```python
from build123d import *

# Parameters (mm, degrees)
SKETCH1_W            = 24.13
SKETCH1_H            = 10.16
BOSS_EXTRUDE1_DEPTH  = 5.334
SKETCH6_W            = 5.334
SKETCH6_H            = 10.16
BOSS_EXTRUDE5_DEPTH  = 5.334
SKETCH11_W           = 5.334
SKETCH11_H           = 10.206206115
BOSS_EXTRUDE6_DEPTH  = 5.334
SKETCH12_W           = 34.798
SKETCH12_H           = 5.334
BOSS_EXTRUDE7_DEPTH  = 5.334
SKETCH13_W           = 5.334
SKETCH13_H           = 0.046206115
CUT_EXTRUDE1_DEPTH   = 32.634561721
SKETCH17_W           = 11.599333333
SKETCH17_H           = 5.334
CUT_EXTRUDE5_DEPTH   = 5.334
SKETCH18_W           = 5.334
SKETCH18_H           = 5.08
SKETCH18_W_2         = 11.684
CUT_EXTRUDE6_DEPTH   = 5.334
SKETCH19_W           = 5.334
SKETCH19_H           = 5.08
BOSS_EXTRUDE8_DEPTH  = 5.334
SKETCH20_W           = 5.334
SKETCH20_H           = 5.08
BOSS_EXTRUDE10_DEPTH = 1.016
SKETCH21_W           = 11.599333334
SKETCH21_H           = 5.334
BOSS_EXTRUDE11_DEPTH = 10.668
SKETCH22_W           = 5.503333334
SKETCH22_H           = 5.334
CUT_EXTRUDE7_DEPTH   = 34.950594339
SKETCH23_W           = 5.334
SKETCH23_H           = 5.08
BOSS_EXTRUDE12_DEPTH = 5.334
SKETCH24_W           = 5.334
SKETCH24_H           = 5.08
CUT_EXTRUDE8_DEPTH   = 5.334
SKETCH25_W           = 5.334
SKETCH25_H           = 5.08
BOSS_EXTRUDE13_DEPTH = 5.334
SKETCH26_W           = 5.334
SKETCH26_H           = 5.08
CUT_EXTRUDE9_DEPTH   = 5.334


with BuildPart() as part:
    # Sketch1 → Boss-Extrude1 (new body)
    with BuildSketch(Plane.XY):
        with Locations((12.065, 5.08)):
            Rectangle(SKETCH1_W, SKETCH1_H)
    extrude(amount=BOSS_EXTRUDE1_DEPTH)

    # Sketch6 → Boss-Extrude5 (add)
    with BuildSketch(Plane(origin=(24.13, 0, 0), x_dir=(0, 0, -1), z_dir=(1, 0, 0))):
        with Locations((-2.667, 5.08)):
            Rectangle(SKETCH6_W, SKETCH6_H)
    extrude(amount=BOSS_EXTRUDE5_DEPTH)

    # Sketch11 → Boss-Extrude6 (add)
    with BuildSketch(Plane.ZY):
        with Locations((2.667, 5.103103058)):
            Rectangle(SKETCH11_W, SKETCH11_H)
    extrude(amount=BOSS_EXTRUDE6_DEPTH)

    # Sketch12 → Boss-Extrude7 (add)
    with BuildSketch(Plane(origin=(0, 0, 0), x_dir=(-1, 0, 0), z_dir=(0, -1, 0))):
        with Locations((-12.065, -2.667)):
            Rectangle(SKETCH12_W, SKETCH12_H)
    extrude(amount=BOSS_EXTRUDE7_DEPTH)

    # Sketch13 → Cut-Extrude1 (cut, through all)
    with BuildSketch(Plane(origin=(0, 0, 0), x_dir=(-1, 0, 0), z_dir=(0, 0, -1))):
        with Locations((2.667, 10.183103058)):
            Rectangle(SKETCH13_W, SKETCH13_H)
    extrude(amount=-CUT_EXTRUDE1_DEPTH, mode=Mode.SUBTRACT)

    # Sketch17 → Cut-Extrude5 (cut)
    with BuildSketch(Plane(origin=(0, -5.334, 0), x_dir=(-1, 0, 0), z_dir=(0, -1, 0))):
        with Locations((-0.465666666, -2.667)):
            Rectangle(SKETCH17_W, SKETCH17_H)
        with Locations((-23.664333334, -2.667)):
            Rectangle(SKETCH17_W, SKETCH17_H)
    extrude(amount=-CUT_EXTRUDE5_DEPTH, mode=Mode.SUBTRACT)

    # Sketch18 → Cut-Extrude6 (cut)
    with BuildSketch(Plane.XY.offset(5.334)):
        with Locations((-2.667, 7.62)):
            Rectangle(SKETCH18_W, SKETCH18_H)
        with Locations((23.622, 7.62)):
            Rectangle(SKETCH18_W_2, SKETCH18_H)
    extrude(amount=-CUT_EXTRUDE6_DEPTH, mode=Mode.SUBTRACT)

    # Sketch19 → Boss-Extrude8 (add)
    with BuildSketch(Plane(origin=(17.78, 0, 0), x_dir=(0, 0, -1), z_dir=(1, 0, 0))):
        with Locations((-2.667, 7.62)):
            Rectangle(SKETCH19_W, SKETCH19_H)
    extrude(amount=BOSS_EXTRUDE8_DEPTH)

    # Sketch20 → Boss-Extrude10 (add)
    with BuildSketch(Plane(origin=(23.114, 0, 0), x_dir=(0, 0, -1), z_dir=(1, 0, 0))):
        with Locations((-2.667, 7.62)):
            Rectangle(SKETCH20_W, SKETCH20_H)
    extrude(amount=BOSS_EXTRUDE10_DEPTH)

    # Sketch21 → Boss-Extrude11 (add)
    with BuildSketch(Plane.XZ.offset(5.334)):
        with Locations((12.065, 2.667)):
            Rectangle(SKETCH21_W, SKETCH21_H)
    extrude(amount=BOSS_EXTRUDE11_DEPTH)

    # Sketch22 → Cut-Extrude7 (cut, through all)
    with BuildSketch(Plane.XY.offset(5.334)):
        with Locations((12.065, -8.001)):
            Rectangle(SKETCH22_W, SKETCH22_H)
    extrude(amount=-CUT_EXTRUDE7_DEPTH, mode=Mode.SUBTRACT)

    # Sketch23 → Boss-Extrude12 (add)
    with BuildSketch(Plane.ZY):
        with Locations((2.667, 7.62)):
            Rectangle(SKETCH23_W, SKETCH23_H)
    extrude(amount=BOSS_EXTRUDE12_DEPTH)

    # Sketch24 → Cut-Extrude8 (cut)
    with BuildSketch(Plane.ZY.offset(5.334)):
        with Locations((2.667, 2.54)):
            Rectangle(SKETCH24_W, SKETCH24_H)
    extrude(amount=-CUT_EXTRUDE8_DEPTH, mode=Mode.SUBTRACT)

    # Sketch25 → Boss-Extrude13 (add)
    with BuildSketch(Plane(origin=(24.13, 0, 0), x_dir=(0, 0, -1), z_dir=(1, 0, 0))):
        with Locations((-2.667, 7.62)):
            Rectangle(SKETCH25_W, SKETCH25_H)
    extrude(amount=BOSS_EXTRUDE13_DEPTH)

    # Sketch26 → Cut-Extrude9 (cut)
    with BuildSketch(Plane(origin=(29.464, 0, 0), x_dir=(0, 0, -1), z_dir=(1, 0, 0))):
        with Locations((-2.667, 2.54)):
            Rectangle(SKETCH26_W, SKETCH26_H)
    extrude(amount=-CUT_EXTRUDE9_DEPTH, mode=Mode.SUBTRACT)


solid = part.part
```
Part model, mm, in its own coordinate system. A direction names the side the tool comes from. Give positions to 0.01 mm unless a question says otherwise; leave off trailing zeros. Loops run counter-clockwise (first coordinate to the right, second up) from the corner with the lowest first, then second, coordinate; pieces in that order, holes last. Notation, with made-up numbers: M 2,32 L 55,32 A21 cw 55,36 Z; hole C -20.5,22 d9. An arc over 180 degrees is marked long. Return JSON: item names as keys, results as strings.
1) 3-axis set-ups, long thin cutter, end or side, ignore diameter. For faces 1 (the face through (9.313, -8, 3)), 2 (the face through (17.865, -8, 3)), 3 (the face through (6.265, -8, 3)): which of +Z, -Z, +X, -X, +Y, -Y reach the whole face in a straight line?
Calculated:
{"face 1": "+Z, -Z", "face 2": "+Z, -Z, +X, -Y", "face 3": "+Z, -Z, -X, -Y"}
2) Drill centre lines: line 1 (X direction, y = -7.5, z = 3); line 2 (Y direction, x = 4.5, z = 1.55); line 3 (X direction, y = -0.75, z = 4.6). Where is each one in solid material? Low to high.
Calculated:
{"line 1": "x = 6.27 to 9.31, 14.82 to 17.86", "line 2": "y = 0 to 10.16", "line 3": "x = 6.27 to 17.86"}
3) Saw through at B-B, the plane y = -8.75. List the corners of the cut face in (x, z), then the cut area to 3 significant figures.
Calculated:
{"outline": "M 6.27,0 L 9.31,0 L 9.31,5.33 L 6.27,5.33 Z; M 14.82,0 L 17.86,0 L 17.86,5.33 L 14.82,5.33 Z", "area": "32.5 mm2"}
4) Saw through at C-C, the plane z = 1.6. List the corners of the cut face in (x, y), then the cut area to 3 significant figures.
Calculated:
{"outline": "M -5.33,5.08 L 0,5.08 L 0,0 L 6.27,0 L 6.27,-16 L 17.86,-16 L 17.86,0 L 24.13,0 L 24.13,5.08 L 29.46,5.08 L 29.46,10.16 L -5.33,10.16 Z; hole M 9.31,-10.67 L 14.82,-10.67 L 14.82,-5.33 L 9.31,-5.33 Z", "area": "456 mm2"}
5) Saw through at A-A, the plane x = 10. List the corners of the cut face in (y, z), then the cut area to 3 significant figures.
Calculated:
{"outline": "M -16,0 L -10.67,0 L -10.67,5.33 L -16,5.33 Z; M -5.33,0 L 10.16,0 L 10.16,5.33 L -5.33,5.33 Z", "area": "111 mm2"}
6) Flat gauge pins, fed straight in: pin 1 Ø1.6 at (x, z) = (-2.5, 3) entering from -Y; pin 2 Ø2.5 at (y, z) = (-4.5, 3.5) entering from -X; pin 3 Ø2.5 at (y, z) = (3.5, 3.5) entering from +X. Where does each tip first touch, or does it go through?
Calculated:
{"pin 1": "stops at y = 5.08", "pin 2": "stops at x = 6.27", "pin 3": "stops at x = 24.13"}
7) Saw through at D-D, the plane x = 5. List the corners of the cut face in (y, z).
Calculated:
{"outline": "M 0,0 L 10.16,0 L 10.16,5.33 L 0,5.33 Z"}
8) Pull direction Y, two halves, no side cores. Call faces 4 (the face through (12, -10.668, 3)), 5 (the face through (12, 0, 5.334)), 6 (the face through (-3, 5.08, 3)): released by +Y, released by -Y, zero draft, split by the parting line, or undercut.
Calculated:
{"face 4": "undercut", "face 5": "zero draft", "face 6": "released by -Y"}
